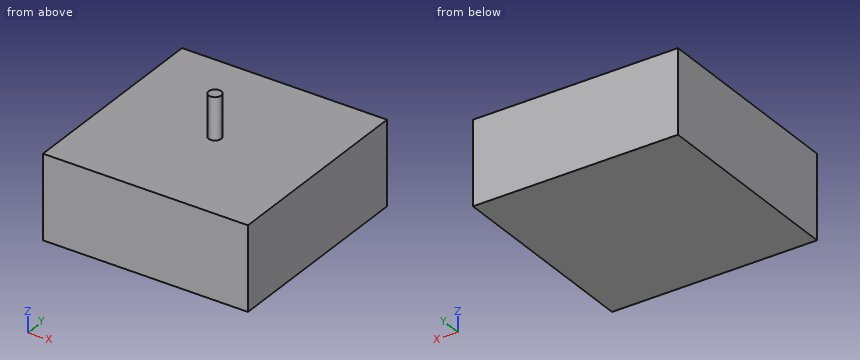
Autodesk Inventor part; units mm, degrees
ref_plane "YZ Plane" through (0, 0, 0) normal (1, 0, 0) x (0, 1, 0)
ref_plane "XZ Plane" through (0, 0, 0) normal (0, 1, 0) x (-1, 0, 0)
ref_plane "XY Plane" through (0, 0, 0) normal (0, 0, 1) x (1, 0, 0)
sketch "Sketch1" plane through (0, 0, 0) normal (0, 0, 1) x (1, 0, 0)
  line L0 (0, 0) -> (49, 0)
  line L1 (49, 0) -> (49, 49)
  line L2 (49, 49) -> (0, 49)
  line L3 (0, 49) -> (0, 0)
  dimension "d0" = 49
  dimension "d1" = 49
extrude "Extrusion1" add sketch "Sketch1" along normal blind 20
sketch "Sketch2" plane through (0, 0, 20) normal (0, 0, 1) x (1, 0, 0)
  circle A0 centre (24.5, 24.5) radius 1.5
  line L0 (49, 49) -> (0, 49)
  line L1 (0, 0) -> (49, 0)
  line L2 (49, 0) -> (49, 49)
  line L3 (0, 49) -> (0, 0)
  dimension "d4" = 3
  dimension "d5" = 49
  dimension "d6" = 49
  dimension "d7" = 24.5
  dimension "d8" = 24.5
extrude "Extrusion2" add sketch "Sketch2" along normal blind 10 contours A0
equation "\"d7\" = 0.5 * d6"
equation "\"d8\" = 0.5 * d5"
properties part number "moteur"
Work out the finished part from the listing and answer in its coordinate system (mm). Round coordinates to 2 decimals unless told otherwise and drop trailing zeros. Order: outer loops, then holes, each group sorted by start corner. A loop starts at its lowest first (then second) coordinate and runs counter-clockwise, first axis right, second up. Notation, with made-up numbers: M -9.75,46.5 L 33.25,46.5 A15 cw 33.25,70.5 Z; hole C -36.5,79 d10. An arc over 180 degrees is marked long. Put each result on its own line as item: value. Start each with the question number.
Q1. Section D-D, the plane y = 44.5 is taken. Write down the section's boundary in (x, z).
Q2. Section A-A, the plane x = 24.5 is taken. Write down the section's boundary in (y, z).
Q3. Section C-C, the plane z = 27.25 is taken. Write down the section's boundary in (x, y), and give its area (3 significant figures).
Q4. A straight line is drawn through the part: L1, parallel to Z at x = 27.5, y = 41.5. Find the intervals that lie inside material, in ascending order. Write a range as [from, to].
Findings below:
1. outline: M 0,0 L 49,0 L 49,20 L 0,20 Z
2. outline: M 0,0 L 49,0 L 49,20 L 26,20 L 26,30 L 23,30 L 23,20 L 0,20 Z
3. outline: C 24.5,24.5 d3
3. area: 7.07 mm^2
4. L1: z = [0, 20]
